```python
from build123d import *

# Parameters (mm, degrees)
PROFILE_SKETCH_W                                = 63.6
PROFILE_SKETCH_H                                = 34.8
PROFILE_EXTRUDE_DEPTH                           = 3.175
MOUNTING_HOLE_SKETCH_R                          = 1.575
MOUNTING_HOLE_CUT_DEPTH                         = 4.175
CSK_FOR_M3_FLAT_HEAD_MACHINE_SCREW1_D           = 3.4
CSK_FOR_M3_FLAT_HEAD_MACHINE_SCREW1_CSINK_D     = 6.3
CSK_FOR_M3_FLAT_HEAD_MACHINE_SCREW1_CSINK_ANGLE = 90
CARRIAGE_GUIDE_HOLE_SKETCH_R                    = 2.1
CARRIAGE_GUIDE_HOLE_CUT_DEPTH                   = 4.175


with BuildPart() as part:
    # Profile Sketch → Profile Extrude (new body)
    with BuildSketch(Plane.XY):
        Rectangle(PROFILE_SKETCH_W, PROFILE_SKETCH_H)
    extrude(amount=PROFILE_EXTRUDE_DEPTH)

    # Mounting Hole Sketch → Mounting Hole Cut (cut, through all)
    with BuildSketch(Plane.XY.offset(3.175)):
        with Locations((-24.3, 12.7)):
            Circle(MOUNTING_HOLE_SKETCH_R)
        with Locations((-24.3, -12.7)):
            Circle(MOUNTING_HOLE_SKETCH_R)
    extrude(amount=-MOUNTING_HOLE_CUT_DEPTH, mode=Mode.SUBTRACT)

    # CSK for M3 Flat Head Machine Screw1 (through all)
    with Locations(Plane(origin=(14.7, 12.7, 3.175), x_dir=(1, 0, 0), z_dir=(0, 0, 1))):
        with Locations((0, 0), (0, -25.4)):
            CounterSinkHole(CSK_FOR_M3_FLAT_HEAD_MACHINE_SCREW1_D / 2, CSK_FOR_M3_FLAT_HEAD_MACHINE_SCREW1_CSINK_D / 2, counter_sink_angle=CSK_FOR_M3_FLAT_HEAD_MACHINE_SCREW1_CSINK_ANGLE)

    # Carriage Guide Hole Sketch → Carriage Guide Hole Cut (cut, through all)
    with BuildSketch(Plane.XY.offset(3.175)):
        with Locations((1.7, 13)):
            Circle(CARRIAGE_GUIDE_HOLE_SKETCH_R)
        with Locations((27.7, 13)):
            Circle(CARRIAGE_GUIDE_HOLE_SKETCH_R)
        with Locations((27.7, -13)):
            Circle(CARRIAGE_GUIDE_HOLE_SKETCH_R)
        with Locations((1.7, -13)):
            Circle(CARRIAGE_GUIDE_HOLE_SKETCH_R)
    extrude(amount=-CARRIAGE_GUIDE_HOLE_CUT_DEPTH, mode=Mode.SUBTRACT)


solid = part.part
```
Check sheet for the modelled part. Datum: model origin and axes. Units: mm. Give positions to 0.01 mm unless a question says otherwise; leave off trailing zeros. Write each loop counter-clockwise with the first axis right and the second up, starting at its lowest first coordinate (ties: lowest second). Pieces come first, ordered by that corner, then holes.
Item 1: Cross-section at A-A (x = -24.3). Enter the section's corners in (y, z) (3 decimals), and give its area (3 significant figures).
Item 2: Cross-section at B-B (z = 0.75). Count the separate pieces of the cut face and the enclosed holes in it, and give its area (3 significant figures).
Item 3: Scan lines: L1, parallel to Y at x = 27.7, z = 1.05; L2, parallel to Y at x = -24.3, z = 0.8 (3 decimals); L3, parallel to X at y = 11.5, z = 1.95. Record each from-to range of solid material in increasing order.
Item 4: Draft check along X on faces 1 (the face through (29.64, 12.2, 1.61)), 2 (the face through (31.8, 0, 2)), 3 (the face through (-31.8, 0, 2)), 4 (the face through (0, -17.4, 2)). Enter one of: released by +X, released by -X, zero draft, split by the parting line, or undercut.
Item 5: Cross-section at C-C (x = 27.7). Enter the section's corners in (y, z) (3 decimals).
Item 6: Gauge pin test, flat ends, axial feed: pin 1 (4 mm diameter, centred on x = 1.7, y = -13, fed in from -Z); pin 2 (4.5 mm diameter, centred on x = 14.7, y = 12.7, fed in from +Z) (3 decimals); pin 3 (5.5 mm diameter, centred on x = 14.7, y = -12.7, fed in from +Z) (3 decimals). Record the tip position at first contact, or that the pin passes through.
Report:
1. outline: (-17.4, 0) - (-14.275, 0) - (-14.275, 3.175) - (-17.4, 3.175) - close; (-11.125, 0) - (11.125, 0) - (11.125, 3.175) - (-11.125, 3.175) - close; (14.275, 0) - (17.4, 0) - (17.4, 3.175) - (14.275, 3.175) - close
1. area: 90.5 mm2
2. separate pieces: 1
2. enclosed holes: 8
2. area: 2,120 mm2
3. L1: y = -17.4 to -15.1, -10.9 to 10.9, 15.1 to 17.4
3. L2: y = -17.4 to -14.275, -11.125 to 11.125, 14.275 to 17.4
3. L3: x = -31.8 to -25.32, -23.28 to 0.23, 3.17 to 13.19, 16.21 to 26.23, 29.17 to 31.8
4. face 1: undercut
4. face 2: released by +X
4. face 3: released by -X
4. face 4: zero draft
5. outline: (-17.4, 0) - (-15.1, 0) - (-15.1, 3.175) - (-17.4, 3.175) - close; (-10.9, 0) - (10.9, 0) - (10.9, 3.175) - (-10.9, 3.175) - close; (15.1, 0) - (17.4, 0) - (17.4, 3.175) - (15.1, 3.175) - close
6. pin 1: passes through
6. pin 2: stops at z = 2.275
6. pin 3: stops at z = 2.775
